The model under review builds one solid part; all positions refer to its coordinate system, in mm. Face numbers are marked on the shaded views. A direction names the side the tool comes from. Coordinates: 2 decimals unless noted, no trailing zeros. Loops run counter-clockwise (first coordinate to the right, second up) from the corner with the lowest first, then second, coordinate; pieces in that order, holes last. Notation, with made-up numbers: (71, 44) - (110, 44) arc R28 cw to (110, 67) - close; hole circle Ø7 at (64.25, 35.5). An arc over 180 degrees is marked (long way). Use a Markdown table: item, result. Add a question column.
1) Add section C-C, the plane z = 2.5. Give the boundary of the cut face in (x, y) (3 decimals).
2) Clearance check with flat-ended pins moving along their axes: pin 1 (2 mm diameter, centred on y = 11, z = 1.5, fed in from +X); pin 2 (2 mm diameter, centred on x = -3, z = 6, fed in from +Y). State where each tip first meets the part, or that it passes through.
3) To check wall thickness, follow L1, parallel to Y at x = 0, z = 6.25; L2, parallel to Z at x = 9.25, y = -2.5; L3, parallel to Y at x = 0, z = 2.75. State the ranges of each line that lie inside material, in increasing order. Write a range as [from, to].
4) Add section A-A, the plane x = 0. Give the boundary of the cut face in (y, z).
5) Add section D-D, the plane z = 5.25. Give the boundary of the cut face in (x, y), and give its area (3 significant figures).
6) Add section B-B, the plane y = 0. Give the boundary of the cut face in (x, z) (3 decimals).
7) The part is to be moulded in two halves that separate along X. For the marked faces 1, 2 and 3, say which applies: pulls with the +X half, pulls with the -X half, needs draft (parallel to the pull), parting line crosses it, or undercut.
8) For the marked faces 4 and 5, list the 3-axis set-ups (+Z, -Z, +X, -X, +Y, -Y) from which the entire face can be reached by the end or side of a thin tool; tool diameter is ignored.
```python
from build123d import *

# Parameters (mm, degrees)
SKETCH_R      = 4
PAD_DEPTH     = 4
SKETCH001_R   = 6.5
SKETCH001_R_2 = 4
PAD001_DEPTH  = 4.8
CHAMFER_SIZE  = 0.5
FILLET_R      = 3
FILLET001_R   = 0.5


with BuildPart() as part:
    # Sketch → Pad (new body)
    with BuildSketch(Plane.XY):
        Polygon((0, 16.36788), (-14.175, 8.18394), (-14.175, -8.18394), (0, -16.36788), (14.175, -8.18394), (14.175, 8.18394), align=None)
        Circle(SKETCH_R, mode=Mode.SUBTRACT)
    extrude(amount=PAD_DEPTH)

    # Sketch001 (on Face9 of Pad) → Pad001 (join)
    with BuildSketch(Plane.XY.offset(4)):
        Circle(SKETCH001_R)
        Circle(SKETCH001_R_2, mode=Mode.SUBTRACT)
    extrude(amount=PAD001_DEPTH)

    # Chamfer
    chamfer_edges = [part.edges().sort_by_distance(p)[0] for p in [
        (-4, 0, 8.8),
    ]]
    chamfer(chamfer_edges, length=CHAMFER_SIZE)

    # Fillet
    fillet_edges = [part.edges().sort_by_distance(p)[0] for p in [
        (0, -16.36788, 2),
        (14.175, -8.18394, 2),
        (14.175, 8.18394, 2),
        (-14.175, -8.18394, 2),
        (-14.175, 8.18394, 2),
        (0, 16.36788, 2),
    ]]
    fillet(fillet_edges, radius=FILLET_R)

    # Fillet001
    fillet001_edges = [part.edges().sort_by_distance(p)[0] for p in [
        (13.773076, -7.951889, 0),
        (7.0875, -12.27591, 0),
        (-7.0875, -12.27591, 0),
        (-13.773076, -7.951889, 0),
        (-14.175, 0, 0),
        (-13.773076, 7.951889, 0),
        (-7.0875, 12.27591, 0),
        (0, 15.903779, 0),
        (7.0875, 12.27591, 0),
        (13.773076, 7.951889, 0),
        (14.175, 0, 0),
        (0, -15.903779, 0),
    ]]
    fillet(fillet001_edges, radius=FILLET001_R)


solid = part.part
```
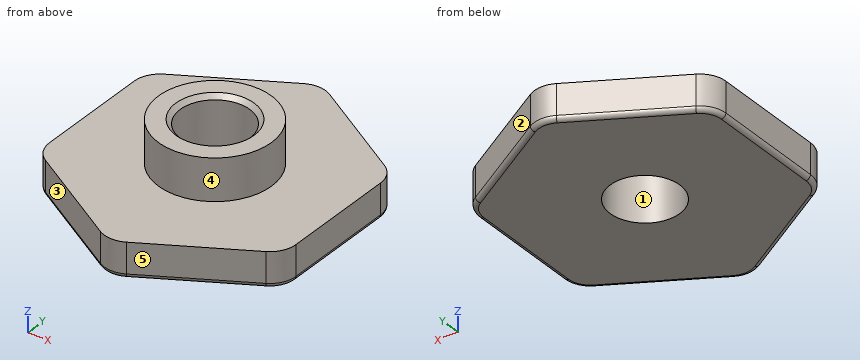
From the geometry:
| question | item | result |
|---|---|---|
| 1 | outline | (-14.175, -6.452) arc R3 ccw to (-12.675, -9.05) - (-1.5, -15.502) arc R3 ccw to (1.5, -15.502) - (12.675, -9.05) arc R3 ccw to (14.175, -6.452) - (14.175, 6.452) arc R3 ccw to (12.675, 9.05) - (1.5, 15.502) arc R3 ccw to (-1.5, 15.502) - (-12.675, 9.05) arc R3 ccw to (-14.175, 6.452) - close; hole circle Ø8 at (0, 0) |
| 2 | pin 1 | stops at x = 11.03 |
| 2 | pin 2 | stops at y = 6.18 |
| 3 | L1 | y = [-6.5, -4], [4, 6.5] |
| 3 | L2 | z = [0, 4] |
| 3 | L3 | y = [-15.9, -4], [4, 15.9] |
| 4 | outline | (-15.9, 0.5) arc R0.5 ccw to (-15.4, 0) - (-4, 0) - (-4, 8.3) - (-4.5, 8.8) - (-6.5, 8.8) - (-6.5, 4) - (-15.9, 4) - close; (4, 0) - (15.4, 0) arc R0.5 ccw to (15.9, 0.5) - (15.9, 4) - (6.5, 4) - (6.5, 8.8) - (4.5, 8.8) - (4, 8.3) - close |
| 5 | outline | circle Ø13 at (0, 0); hole circle Ø8 at (0, 0) |
| 5 | area | 82.5 mm^2 |
| 6 | outline | (-14.175, 0.5) arc R0.5 ccw to (-13.675, 0) - (-4, 0) - (-4, 8.3) - (-4.5, 8.8) - (-6.5, 8.8) - (-6.5, 4) - (-14.175, 4) - close; (4, 0) - (13.675, 0) arc R0.5 ccw to (14.175, 0.5) - (14.175, 4) - (6.5, 4) - (6.5, 8.8) - (4.5, 8.8) - (4, 8.3) - close |
| 7 | face 1 | undercut |
| 7 | face 2 | pulls with the +X half |
| 7 | face 3 | pulls with the -X half |
| 8 | face 4 | +Z |
| 8 | face 5 | +Z, -Z, +X, -Y |
